Check sheet for the modelled part. Datum: model origin and axes. Units: mm. A direction names the side the tool comes from. Round coordinates to 2 decimals unless told otherwise and drop trailing zeros. Order: outer loops, then holes, each group sorted by start corner. A loop starts at its lowest first (then second) coordinate and runs counter-clockwise, first axis right, second up. Notation, with made-up numbers: M 82.25,-13.5 L 118.25,-13.5 A10 cw 118.25,-7.5 Z; hole C 48,75 d10. An arc over 180 degrees is marked long. One line per item, written item: value. Start each with the question number.
(1) Cross-section at C-C, the plane y = 1.75. Enter the section's corners in (x, z).
(2) Thickness scan on L1, parallel to X at y = 6.25, z = 27; L2, parallel to X at y = -1, z = 11; L3, parallel to X at y = -1.75, z = 5.5. Record the ranges inside material, lowest first.
(3) Depth check by flat-ended pin: pin 1 Ø4 at (x, y) = (3, -6.5) entering from +Z; pin 2 Ø1 at (y, z) = (-2, 11) entering from -X; pin 3 Ø5 at (y, z) = (-3.5, 38) entering from -X. Enter the tip coordinate at first touch or a pass-through.
(4) Cross-section at A-A, the plane z = 30. Enter the section's corners in (x, y).
(5) Access from +Z, -Z, +X, -X, +Y, -Y to the whole of each face (thin tool, end or side, straight path). Record for faces 1 (the face through (6, -8.539, 17)), 2 (the face through (7.878, 0, 32)), 3 (the face through (-1, -11, 13.208)).
(6) Cross-section at D-D, the plane x = 0. Enter the section's corners in (y, z), and give its area (3 significant figures).
(7) Cross-section at B-B, the plane x = -12. Enter the section's corners in (y, z).
(8) Release check for a two-part mould opening along X. For faces 4 (the face through (-25.4, 0, 29)), 5 (the face through (-1, -12.521, 7)), 6 (the face through (25.4, 0, 29)), 7 (the face through (-0.173, 0.12, 16.226)) record: released by +X, released by -X, zero draft, split by the parting line, or undercut.
from build123d import *

# Parameters (mm, degrees)
F1_DEPTH = 13.208
F3_DEPTH = 25.4
F4_DEPTH = 25.4
F6_DEPTH = 25.4
F7_DEPTH = 25.4


with BuildPart() as f1:
    # F0 (on Top) → F1 (new body)
    with BuildSketch(Plane.XY):
        with BuildLine():
            ThreePointArc((39.5257622004, -12.5212473795), (27.0045148209, 0), (39.5257622004, 12.5212473795))
            Line((39.5257622004, 12.5212473795), (-39.5257622004, 12.5212473795))
            ThreePointArc((-39.5257622004, 12.5212473795), (-30.6719032694, 8.8538589309), (-27.0045148209, 0))
            ThreePointArc((-27.0045148209, 0), (-30.6719032694, -8.8538589309), (-39.5257622004, -12.5212473795))
            Line((-39.5257622004, -12.5212473795), (39.5257622004, -12.5212473795))
        make_face()
        with BuildLine():
            ThreePointArc((52.0470095798, 0), (48.3796211313, 8.8538589309), (39.5257622004, 12.5212473795))
            Line((39.5257622004, 12.5212473795), (39.5257622004, 6.073428591))
            ThreePointArc((39.5257622004, 6.073428591), (43.8203247421, 4.2945625417), (45.5991907913, 0))
            ThreePointArc((45.5991907913, 0), (43.8203247421, -4.2945625417), (39.5257622004, -6.073428591))
            Line((39.5257622004, -6.073428591), (39.5257622004, -12.5212473795))
            ThreePointArc((39.5257622004, -12.5212473795), (48.3796211313, -8.8538589309), (52.0470095798, 0))
        make_face()
        with BuildLine():
            Line((39.5257622004, 6.073428591), (39.5257622004, 12.5212473795))
            ThreePointArc((39.5257622004, 12.5212473795), (27.0045148209, 0), (39.5257622004, -12.5212473795))
            Line((39.5257622004, -12.5212473795), (39.5257622004, -6.073428591))
            ThreePointArc((39.5257622004, -6.073428591), (33.4523336094, 0), (39.5257622004, 6.073428591))
        make_face()
        with BuildLine():
            ThreePointArc((-27.0045148209, 0), (-30.6719032694, 8.8538589309), (-39.5257622004, 12.5212473795))
            Line((-39.5257622004, 12.5212473795), (-39.5257622004, 6.073428591))
            ThreePointArc((-39.5257622004, 6.073428591), (-35.2311996586, 4.2945625417), (-33.4523336094, 0))
            ThreePointArc((-33.4523336094, 0), (-35.2311996586, -4.2945625417), (-39.5257622004, -6.073428591))
            Line((-39.5257622004, -6.073428591), (-39.5257622004, -12.5212473795))
            ThreePointArc((-39.5257622004, -12.5212473795), (-30.6719032694, -8.8538589309), (-27.0045148209, 0))
        make_face()
        with BuildLine():
            Line((-39.5257622004, 6.073428591), (-39.5257622004, 12.5212473795))
            ThreePointArc((-39.5257622004, 12.5212473795), (-52.0470095798, 0), (-39.5257622004, -12.5212473795))
            Line((-39.5257622004, -12.5212473795), (-39.5257622004, -6.073428591))
            ThreePointArc((-39.5257622004, -6.073428591), (-45.5991907913, 0), (-39.5257622004, 6.073428591))
        make_face()
    extrude(amount=F1_DEPTH)

    # F2 (on Right) → F3 (join)
    with BuildSketch(Plane.YZ):
        with BuildLine():
            Line((8.5389625284, 35.6879048049), (3.3581880853, 35.6879048049))
            ThreePointArc((3.3581880853, 35.6879048049), (0, 32.3297167197), (-3.3581880853, 35.6879048049))
            Line((-3.3581880853, 35.6879048049), (-8.5389625284, 35.6879048049))
            ThreePointArc((-8.5389625284, 35.6879048049), (0, 27.1489422766), (8.5389625284, 35.6879048049))
        make_face()
        with BuildLine():
            ThreePointArc((-3.3581880853, 35.6879048049), (0, 39.0460928902), (3.3581880853, 35.6879048049))
            Line((3.3581880853, 35.6879048049), (8.5389625284, 35.6879048049))
            ThreePointArc((8.5389625284, 35.6879048049), (0, 44.2268673333), (-8.5389625284, 35.6879048049))
            Line((-8.5389625284, 35.6879048049), (-3.3581880853, 35.6879048049))
        make_face()
        with BuildLine():
            Line((8.5389625284, 0), (8.5389625284, 35.6879048049))
            ThreePointArc((8.5389625284, 35.6879048049), (0, 27.1489422766), (-8.5389625284, 35.6879048049))
            Line((-8.5389625284, 35.6879048049), (-8.5389625284, 0))
            Line((-8.5389625284, 0), (8.5389625284, 0))
        make_face()
    extrude(amount=F3_DEPTH)

    # F2 (on Right) → F4 (join)
    with BuildSketch(Plane.YZ):
        with BuildLine():
            Line((8.5389625284, 35.6879048049), (3.3581880853, 35.6879048049))
            ThreePointArc((3.3581880853, 35.6879048049), (0, 32.3297167197), (-3.3581880853, 35.6879048049))
            Line((-3.3581880853, 35.6879048049), (-8.5389625284, 35.6879048049))
            ThreePointArc((-8.5389625284, 35.6879048049), (0, 27.1489422766), (8.5389625284, 35.6879048049))
        make_face()
        with BuildLine():
            ThreePointArc((-3.3581880853, 35.6879048049), (0, 39.0460928902), (3.3581880853, 35.6879048049))
            Line((3.3581880853, 35.6879048049), (8.5389625284, 35.6879048049))
            ThreePointArc((8.5389625284, 35.6879048049), (0, 44.2268673333), (-8.5389625284, 35.6879048049))
            Line((-8.5389625284, 35.6879048049), (-3.3581880853, 35.6879048049))
        make_face()
        with BuildLine():
            Line((8.5389625284, 0), (8.5389625284, 35.6879048049))
            ThreePointArc((8.5389625284, 35.6879048049), (0, 27.1489422766), (-8.5389625284, 35.6879048049))
            Line((-8.5389625284, 35.6879048049), (-8.5389625284, 0))
            Line((-8.5389625284, 0), (8.5389625284, 0))
        make_face()
    extrude(amount=-F4_DEPTH)

    # F5 (on Front) → F6 (cut)
    with BuildSketch(Plane.XZ):
        with BuildLine():
            Line((-7.8779369453, 24.1020768881), (7.8779369453, 24.1020768881))
            ThreePointArc((7.8779369453, 24.1020768881), (0, 31.9800138334), (-7.8779369453, 24.1020768881))
        make_face()
        with BuildLine():
            ThreePointArc((-7.8779369453, 24.1020768881), (0, 16.2241399428), (7.8779369453, 24.1020768881))
            Line((7.8779369453, 24.1020768881), (-7.8779369453, 24.1020768881))
        make_face()
        with BuildLine():
            ThreePointArc((-7.8779369453, 24.1020768881), (0, 31.9800138334), (7.8779369453, 24.1020768881))
            Line((7.8779369453, 24.1020768881), (7.8779369453, 49.5002679527))
            Line((7.8779369453, 49.5002679527), (-7.8779369453, 49.5002679527))
            Line((-7.8779369453, 49.5002679527), (-7.8779369453, 24.1020768881))
        make_face()
    extrude(amount=-F6_DEPTH, mode=Mode.SUBTRACT)

    # F5 (on Front) → F7 (cut)
    with BuildSketch(Plane.XZ):
        with BuildLine():
            Line((-7.8779369453, 24.1020768881), (7.8779369453, 24.1020768881))
            ThreePointArc((7.8779369453, 24.1020768881), (0, 31.9800138334), (-7.8779369453, 24.1020768881))
        make_face()
        with BuildLine():
            ThreePointArc((-7.8779369453, 24.1020768881), (0, 16.2241399428), (7.8779369453, 24.1020768881))
            Line((7.8779369453, 24.1020768881), (-7.8779369453, 24.1020768881))
        make_face()
        with BuildLine():
            ThreePointArc((-7.8779369453, 24.1020768881), (0, 31.9800138334), (7.8779369453, 24.1020768881))
            Line((7.8779369453, 24.1020768881), (7.8779369453, 49.5002679527))
            Line((7.8779369453, 49.5002679527), (-7.8779369453, 49.5002679527))
            Line((-7.8779369453, 49.5002679527), (-7.8779369453, 24.1020768881))
        make_face()
    extrude(amount=F7_DEPTH, mode=Mode.SUBTRACT)


solid = f1.part
Values found:
1. outline: M -51.92,0 L -45.34,0 L -45.34,13.21 L -51.92,13.21 Z; M -33.71,0 L 33.71,0 L 33.71,13.21 L 25.4,13.21 L 25.4,32.82 L 7.88,32.82 L 7.88,24.1 A7.88 cw -7.88,24.1 L -7.88,32.82 L -25.4,32.82 L -25.4,13.21 L -33.71,13.21 Z; M -25.4,38.55 L -7.88,38.55 L -7.88,44.05 L -25.4,44.05 Z; M 7.88,38.55 L 25.4,38.55 L 25.4,44.05 L 7.88,44.05 Z; M 45.34,0 L 51.92,0 L 51.92,13.21 L 45.34,13.21 Z
2. L1: -25.4 to -7.88, 7.88 to 25.4
2. L2: -52.01 to -45.52, -33.54 to 33.54, 45.52 to 52.01
2. L3: -51.92 to -45.34, -33.71 to 33.71, 45.34 to 51.92
3. pin 1: z = 18.01
3. pin 2: x = -51.96
3. pin 3: x = -25.4
4. outline: M -25.4,-8.54 L -7.88,-8.54 L -7.88,8.54 L -25.4,8.54 Z; M 7.88,-8.54 L 25.4,-8.54 L 25.4,8.54 L 7.88,8.54 Z
5. face 1: +Z, +X, -X, -Y
5. face 2: +Z, +Y, -Y
5. face 3: +Z
6. outline: M -12.52,0 L 12.52,0 L 12.52,13.21 L 8.54,13.21 L 8.54,16.22 L -8.54,16.22 L -8.54,13.21 L -12.52,13.21 Z
6. area: 382 mm^2
7. outline: M -12.52,0 L 12.52,0 L 12.52,13.21 L 8.54,13.21 L 8.54,35.69 A8.54 ccw -8.54,35.69 L -8.54,13.21 L -12.52,13.21 Z; hole C 0,35.69 d6.72
8. face 4: released by -X
8. face 5: zero draft
8. face 6: released by +X
8. face 7: undercut
